from build123d import *

# Parameters (mm, degrees)
SKETCH_W        = 48
SKETCH_H        = 72.4
PAD_DEPTH       = 2
FILLET_R        = 1
SKETCH001_W     = 18
SKETCH001_H     = 35
PAD001_DEPTH    = 3
SKETCH002_W     = 14
SKETCH002_H     = 17
POCKET_DEPTH    = 1
SKETCH003_W     = 7
SKETCH003_H     = 4
POCKET001_DEPTH = 1
PAD002_DEPTH    = 2


with BuildPart() as obj1:
    # Sketch → Pad (new body)
    with BuildSketch(Plane.XY):
        Rectangle(SKETCH_W, SKETCH_H)
    extrude(amount=PAD_DEPTH)

    # Fillet
    fillet_edges = [obj1.edges().sort_by_distance(p)[0] for p in [
        (-24, 36.2, 1),
        (24, 36.2, 1),
        (24, -36.2, 1),
        (-24, -36.2, 1),
    ]]
    fillet(fillet_edges, radius=FILLET_R)

    # Sketch001 → Pad001 (new body)
    with BuildSketch(Plane(origin=(0, 0, 0), x_dir=(1, 0, 0), z_dir=(0, 0, -1))):
        Rectangle(SKETCH001_W, SKETCH001_H)
    extrude(amount=PAD001_DEPTH)

    # Sketch002 → Pocket (cut)
    with BuildSketch(Plane(origin=(0, 0, -3), x_dir=(1, 0, 0), z_dir=(0, 0, -1))):
        with Locations((0, -9)):
            Rectangle(SKETCH002_W, SKETCH002_H)
    extrude(amount=-POCKET_DEPTH, mode=Mode.SUBTRACT)

    # Sketch003 → Pocket001 (cut)
    with BuildSketch(Plane(origin=(0, 0, -2), x_dir=(1, 0, 0), z_dir=(0, 0, -1))):
        with Locations((0, -14)):
            Rectangle(SKETCH003_W, SKETCH003_H)
    extrude(amount=-POCKET001_DEPTH, mode=Mode.SUBTRACT)

    # Sketch004 → Pad002 (new body)
    with BuildSketch(Plane.YZ.offset(9)):
        Polygon((15.5, -3), (15.5, -1.5), (-6.5, -1.5), (-6.5, 0), (-17.5, 0), (-17.5, -3), align=None)
    extrude(amount=PAD002_DEPTH)


with BuildPart() as part_mirroring:
    # Part__Mirroring: instance of obj1
    add(obj1.part.mirror(Plane(origin=(0, 0, 0), x_dir=(0, -1, 0), z_dir=(1, 0, 0))))


solid = part_mirroring.part
The model under review builds one solid part; all positions refer to its coordinate system, in mm. A direction names the side the tool comes from. Give positions to 0.01 mm unless a question says otherwise; leave off trailing zeros. Loops run counter-clockwise (first coordinate to the right, second up) from the corner with the lowest first, then second, coordinate; pieces in that order, holes last. Notation, with made-up numbers: (25, -15) -> (48, -15) arc R7 cw to (48, -7) -> close; hole circle Ø4 at (-38, 33.5). An arc over 180 degrees is marked (long way). Answer as a JSON object with one key per item and string values. Group by question number.
Q1. Take a section at A-A (x = -6). Write out the cut boundary in (y, z), plus the area to 3 significant figures.
Q2. Wall thickness on line 1 along Y through (x, z) = (1, -1.15); line 2 along Z through (x, y) = (-20.5, 0); line 3 along Y through (x, z) = (-1.5, -0.9): over which ranges is each line inside the solid? List them lowest first.
Q3. Take a section at C-C (x = 2). Write out the cut boundary in (y, z), plus the area to 3 significant figures.
Q4. Tool access review of faces 1 (the flat face through (-10, 15.5, -2)), 2 (the flat face through (-1, -17.5, -1)), 3 (the flat face through (9, 0, -1)), 4 (the flat face through (0, 9, -2)): name each direction out of +Z, -Z, +X, -X, +Y, -Y from which nothing blocks a thin tool from reaching the whole face with its end or side.
Q5. Draft analysis for pull direction Z (two halves, no side actions). For faces 5 (the flat face through (-10, -6.5, -1)), 6 (the flat face through (-1, -4, -3)), 7 (the flat face through (0, 1, 2)), 8 (the flat face through (-11, -5, -2)), state which applies: pulls with the +Z half, pulls with the -Z half, needs draft (parallel to the pull), parting line crosses it, or undercut.
Q6. Take a section at D-D (y = 5.5). Write out the cut boundary in (x, z), plus the area to 3 significant figures.
Q7. Insertion check: pin 1 (0.8 mm diameter, centred on x = 0, z = -1.5, fed in from -Y); pin 2 (1.1 mm diameter, centred on y = 14.5, z = -1.5, fed in from -X); pin 3 (2 mm diameter, centred on x = 1, y = 14.5, fed in from -Z). Each pin has a flat end and moves straight along its axis. Give the tip position at first contact, or say it passes through.
Q8. Take a section at B-B (y = 13.5). Write out the cut boundary in (x, z), plus the area to 3 significant figures.
Answer below:
{
 "1": {"outline": "(-36.2, 0) -> (-17.5, 0) -> (-17.5, -3) -> (0.5, -3) -> (0.5, -2) -> (17.5, -2) -> (17.5, 0) -> (36.2, 0) -> (36.2, 2) -> (-36.2, 2) -> close", "area": "233 mm2"},
 "2": {"line 1": "y = -17.5 to 12, 16 to 17.5", "line 2": "z = 0 to 2", "line 3": "y = -17.5 to 17.5"},
 "3": {"outline": "(-36.2, 0) -> (-17.5, 0) -> (-17.5, -3) -> (0.5, -3) -> (0.5, -2) -> (12, -2) -> (12, -1) -> (16, -1) -> (16, -2) -> (17.5, -2) -> (17.5, 0) -> (36.2, 0) -> (36.2, 2) -> (-36.2, 2) -> close", "area": "229 mm2"},
 "4": {"face 1": "-Z, -X, +Y", "face 2": "-Z, +X, -X, -Y", "face 3": "-Z, +X, +Y, -Y", "face 4": "-Z, +Y"},
 "5": {"face 5": "undercut", "face 6": "pulls with the -Z half", "face 7": "pulls with the +Z half", "face 8": "needs draft"},
 "6": {"outline": "(-24, 0) -> (-9, 0) -> (-9, -1.5) -> (-11, -1.5) -> (-11, -3) -> (-7, -3) -> (-7, -2) -> (7, -2) -> (7, -3) -> (9, -3) -> (9, 0) -> (24, 0) -> (24, 2) -> (-24, 2) -> close", "area": "139 mm2"},
 "7": {"pin 1": "stops at y = -17.5", "pin 2": "stops at x = -11", "pin 3": "stops at z = -1"},
 "8": {"outline": "(-24, 0) -> (-9, 0) -> (-9, -1.5) -> (-11, -1.5) -> (-11, -3) -> (-7, -3) -> (-7, -2) -> (-3.5, -2) -> (-3.5, -1) -> (3.5, -1) -> (3.5, -2) -> (7, -2) -> (7, -3) -> (9, -3) -> (9, 0) -> (24, 0) -> (24, 2) -> (-24, 2) -> close", "area": "132 mm2"}
}
